```python
from build123d import *

# Parameters (mm, degrees)
F0_R     = 21
F1_DEPTH = 13
F2_R     = 7.5
F3_DEPTH = 37.3
F4_SIZE  = 0.5


with BuildPart() as f1:
    # F0 (on Top) → F1 (new body)
    with BuildSketch(Plane.XY):
        Circle(F0_R)
    extrude(amount=F1_DEPTH)

    # F2 (on face) → F3 (cut)
    with BuildSketch(Plane.XY.offset(13)):
        Circle(F2_R)
    extrude(amount=-F3_DEPTH, mode=Mode.SUBTRACT)

    # F4
    f4_edges = [f1.edges().sort_by_distance(p)[0] for p in [
        (-21, 0, 13),
        (-7.5, 0, 13),
        (-21, 0, 0),
        (-7.5, 0, 0),
    ]]
    chamfer(f4_edges, length=F4_SIZE)


solid = f1.part
```
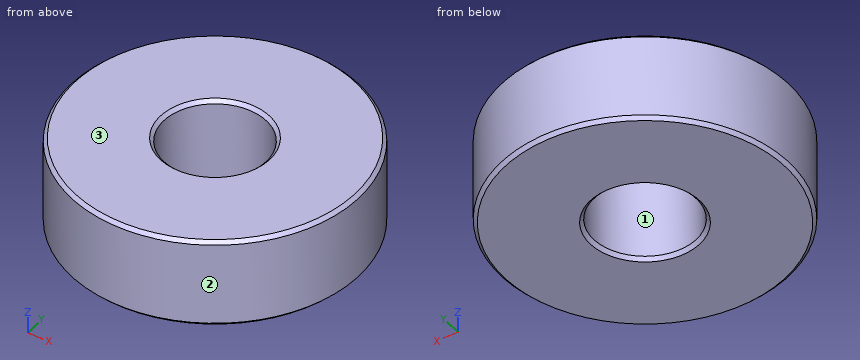
Build history of the part. All positions in model axes, mm. Face numbers are marked on the shaded views. Coordinates: 2 decimals unless noted, no trailing zeros. Order: outer loops, then holes, each group sorted by start corner. A loop starts at its lowest first (then second) coordinate and runs counter-clockwise, first axis right, second up.
Item 1: Drill centre lines: L1, parallel to Y at x = 0, z = 9; L2, parallel to Y at x = -5, z = 6; L3, parallel to X at y = -4, z = 3.5. Where is each one in solid material? Low to high.
Filled in:
L1: y = -21 to -7.5, 7.5 to 21
L2: y = -20.4 to -5.59, 5.59 to 20.4
L3: x = -20.62 to -6.34, 6.34 to 20.62
Item 2: Saw through at A-A on x = 0. List the corners of the cut face in (y, z).
Filled in:
outline: (-21, 0.5) - (-20.5, 0) - (-8, 0) - (-7.5, 0.5) - (-7.5, 12.5) - (-8, 13) - (-20.5, 13) - (-21, 12.5) - close; (7.5, 0.5) - (8, 0) - (20.5, 0) - (21, 0.5) - (21, 12.5) - (20.5, 13) - (8, 13) - (7.5, 12.5) - close
Item 3: Saw through at C-C on z = 2.75. List the corners of the cut face in (x, y).
Filled in:
outline: circle Ø42 at (0, 0); hole circle Ø15 at (0, 0)
Item 4: Mould opens along Y. For the marked faces 1, 2 and 3 say: released by +Y, released by -Y, zero draft, split by the parting line, or undercut.
Filled in:
face 1: undercut
face 2: split by the parting line
face 3: zero draft
Item 5: Drop flat-ended pins along their axis: pin 1 Ø2 at (x, z) = (10.5, 10.5) entering from -Y; pin 2 Ø6 at (x, z) = (-14.5, 6) entering from +Y; pin 3 Ø1 at (y, z) = (10, 9.5) entering from -X. Give the stop position or say it passes through.
Filled in:
pin 1: stops at y = -18.73
pin 2: stops at y = 17.57
pin 3: stops at x = -18.73
